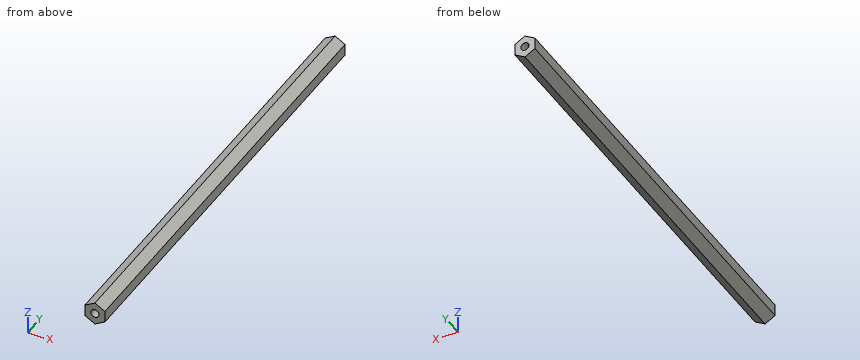
Autodesk Inventor part; units mm, degrees
ref_plane "YZ Plane" through (0, 0, 0) normal (1, 0, 0) x (0, 1, 0)
ref_plane "XZ Plane" through (0, 0, 0) normal (0, 1, 0) x (-1, 0, 0)
ref_plane "XY Plane" through (0, 0, 0) normal (0, 0, 1) x (1, 0, 0)
sketch "Sketch1" plane through (0, 0, 0) normal (0, 1, 0) x (-1, 0, 0)
  line L0 (-6.35, -3.6662) -> (-6.35, 3.6662)
  line L1 (-6.35, 3.6662) -> (0, 7.3323)
  line L2 (0, 7.3323) -> (6.35, 3.6662)
  line L3 (6.35, 3.6662) -> (6.35, -3.6662)
  line L4 (6.35, -3.6662) -> (0, -7.3323)
  line L5 (0, -7.3323) -> (-6.35, -3.6662)
  point P0 (0, 0)
  point P1 (0, 0)
  dimension "d0" = 12.7
extrude "Extrusion1" add sketch "Sketch1" along normal blind 282.575
sketch "Sketch2" plane through (0, 282.575, 0) normal (0, 1, 0) x (1, 0, 0)
  circle A0 centre (0, 0) radius 2.5527
  dimension "d4" = 5.1054
extrude "Extrusion2" cut sketch "Sketch2" against normal blind 25.4
sketch "Sketch3" plane through (0, 0, 0) normal (0, -1, 0) x (1, 0, 0)
  circle A0 centre (0, 0) radius 2.5527
  dimension "d7" = 5.1054
extrude "Extrusion3" cut sketch "Sketch3" against normal blind 25.4
properties part number "INDX_018_FeedFrontHex" material "Aluminum 6061"
Model file for the job. Use its own axes, mm. Coordinates: 2 decimals unless noted, no trailing zeros. Write each loop counter-clockwise with the first axis right and the second up, starting at its lowest first coordinate (ties: lowest second). Pieces come first, ordered by that corner, then holes. Notation, with made-up numbers: (37.5, 43.5) - (41.5, 43.5) arc R18 cw to (41.5, 74.5) - close; hole circle Ø10 at (81, -18). An arc over 180 degrees is marked (long way). Use a Markdown table: item, result. Add a question column.
Item 1: Drop flat-ended pins along their axis: pin 1 (3 mm diameter, centred on x = 0, z = 0, fed in from -Y); pin 2 (6 mm diameter, centred on x = -4.5, y = 105, fed in from -Z); pin 3 (5 mm diameter, centred on x = 5, y = 199, fed in from +Z). Give the stop position or say it passes through.
Item 2: Band-saw the part on B-B, the plane y = 184.5. Write the cut outline in (x, z).
Item 3: Band-saw the part on A-A, the plane z = 0. Write the cut outline in (x, y) (3 decimals), and give its area (3 significant figures).
Item 4: Drill centre lines: line 1 along X through (y, z) = (269, 0); line 2 along Z through (x, y) = (0, 276.5); line 3 along Z through (x, y) = (-2, 14). Where is each one in solid material? Low to high.
A:
| question | item | result |
|---|---|---|
| 1 | pin 1 | stops at y = 25.4 |
| 1 | pin 2 | stops at z = -6.47 |
| 1 | pin 3 | stops at z = 5.89 |
| 2 | outline | (-6.35, -3.67) - (0, -7.33) - (6.35, -3.67) - (6.35, 3.67) - (0, 7.33) - (-6.35, 3.67) - close |
| 3 | outline | (-6.35, 0) - (-2.553, 0) - (-2.553, 25.4) - (2.553, 25.4) - (2.553, 0) - (6.35, 0) - (6.35, 282.575) - (2.553, 282.575) - (2.553, 257.175) - (-2.553, 257.175) - (-2.553, 282.575) - (-6.35, 282.575) - close |
| 3 | area | 3,330 mm² |
| 4 | line 1 | x = -6.35 to -2.55, 2.55 to 6.35 |
| 4 | line 2 | z = -7.33 to -2.55, 2.55 to 7.33 |
| 4 | line 3 | z = -6.18 to -1.59, 1.59 to 6.18 |
